Build history of the part. All positions in model axes, mm. Round coordinates to 2 decimals unless told otherwise and drop trailing zeros. Write each loop counter-clockwise with the first axis right and the second up, starting at its lowest first coordinate (ties: lowest second). Pieces come first, ordered by that corner, then holes. Notation, with made-up numbers: (-6.75, 69.5) - (11.25, 69.5) arc R17 cw to (11.25, 98.5) - close; hole circle Ø9 at (-2, 6.25). An arc over 180 degrees is marked (long way). Answer as a JSON object with one key per item and string values. Group by question number.
Item 1: Probe line 1 (Y direction, x = -2, z = -0.1); line 2 (Y direction, x = -0.75, z = 2); line 3 (X direction, y = 14.25, z = -0.8). List the from-to ranges inside material, lowest first. Write a range as from..to.
Item 2: Slice it at D-D, the plane z = -1.95. List the corners of the cut face in (x, y).
Item 3: Slice it at C-C, the plane y = 16. List the corners of the cut face in (x, z), then the cut area to 3 significant figures.
Item 4: Slice it at B-B, the plane z = -0.15. List the corners of the cut face in (x, y), then the cut area to 3 significant figures.
Item 5: Flat gauge pin, fed straight in: pin 1 (1.5 mm diameter, centred on y = 16, z = 1, fed in from -X). Where does the tip first touch, or does it go through?
Item 6: Two-plate mould, pull along X, no slides. Class faces 1 (the flat face through (0, 10, -2.5)), 2 (the flat face through (11, 6, 0)), 3 (the flat face through (-11, 7, 0)): +X half, -X half, draft (parallel to the pull), parting line (faces both ways), or undercut.
Item 7: Slice it at A-A, the plane x = -4.5. List the corners of the cut face in (y, z) (3 decimals), then the cut area to 3 significant figures.
Autodesk Inventor part; units mm, degrees
ref_plane "YZ Plane" through (0, 0, 0) normal (1, 0, 0) x (0, 1, 0)
ref_plane "XZ Plane" through (0, 0, 0) normal (0, 1, 0) x (-1, 0, 0)
ref_plane "XY Plane" through (0, 0, 0) normal (0, 0, 1) x (1, 0, 0)
sketch "Sketch1" plane through (0, 0, 0) normal (0, 0, 1) x (1, 0, 0)
  line L0 (-11, 0) -> (11, 0)
  line L1 (11, 0) -> (11, 19)
  line L2 (11, 19) -> (-11, 19)
  line L3 (-11, 19) -> (-11, 0)
  point P0 (0, 0)
  point P1 (0, 0)
  dimension "d0" = 22
  dimension "d1" = 19
extrude "Extrusion1" add sketch "Sketch1" along normal mid plane 5
chamfer "Chamfer1" distance 6 angle 45 2 edges at (-11, 19, 0) (11, 19, 0)
sketch "Sketch2" plane through (11, 0, 2.5) normal (1, 0, 0) x (0, 0, -1)
  line L0 (0, 0) -> (0, 13)
  line L1 (5, 13) -> (5, 0)
  arc A0 (0, 1) -> (5, 1) centre (2.5, 3.625) ccw
  line L2 (0, 0) -> (5, 0)
  point P0 (2.5, 0)
  point P1 (2.5, 0)
  dimension "d7" = 1
extrude "Extrusion2" cut sketch "Sketch2" against normal through all
properties material "Steel"
Geometry says:
{
 "1": {"line 1": "y = 0..19", "line 2": "y = 0.6..19", "line 3": "x = -9.75..9.75"},
 "2": {"outline": "(-11, 0.57) - (11, 0.57) - (11, 13) - (5, 19) - (-5, 19) - (-11, 13) - close"},
 "3": {"outline": "(-8, -2.5) - (8, -2.5) - (8, 2.5) - (-8, 2.5) - close", "area": "80.0 mm^2"},
 "4": {"outline": "(-11, 0) - (11, 0) - (11, 13) - (5, 19) - (-5, 19) - (-11, 13) - close", "area": "382 mm^2"},
 "5": {"pin 1": "stops at x = -8.75"},
 "6": {"face 1": "draft", "face 2": "+X half", "face 3": "-X half"},
 "7": {"outline": "(1, -2.5) - (19, -2.5) - (19, 2.5) - (1, 2.5) arc R3.625 ccw to start", "area": "93.4 mm^2"}
}
